Answer from the drawing. Dimensions are ordinates in mm from the lowest x, y and z of the part. A direction names the side the tool comes from. Give positions to 0.01 mm unless a question says otherwise; leave off trailing zeros. Loops run counter-clockwise (first coordinate to the right, second up) from the corner with the lowest first, then second, coordinate; pieces in that order, holes last.
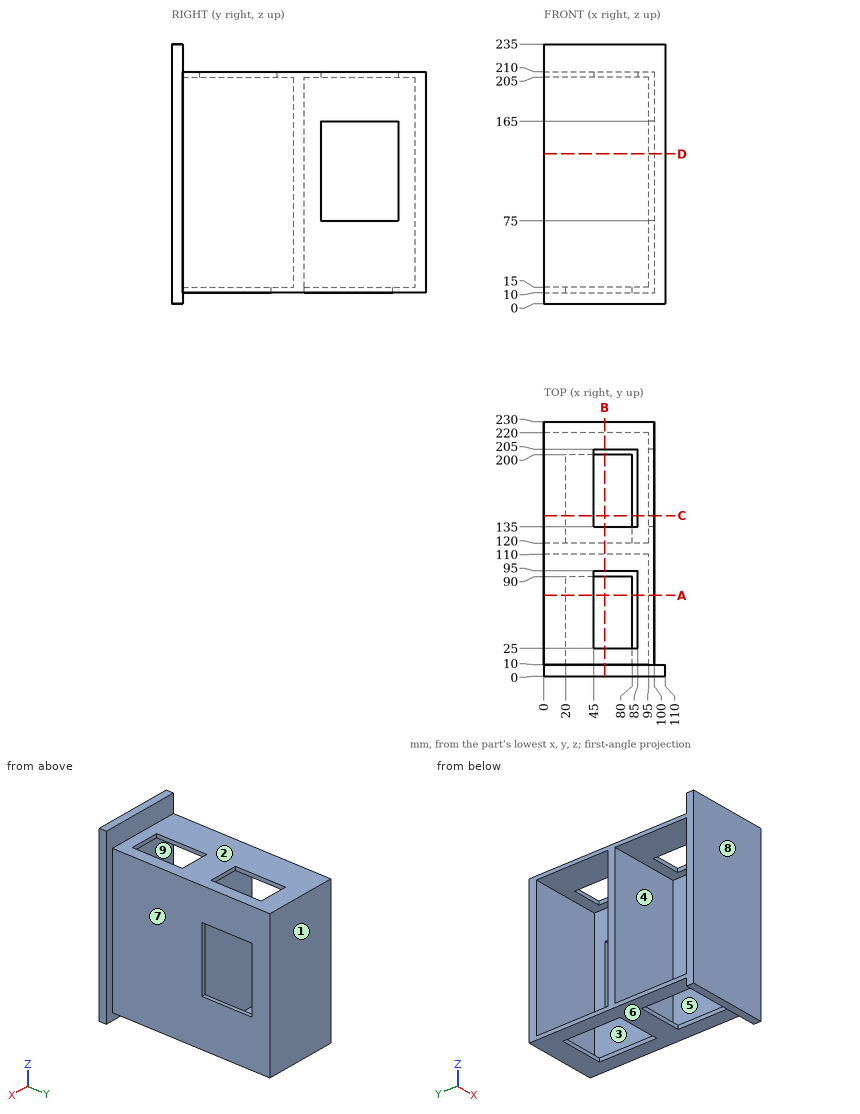
Item 1: Find section C-C, the plane y = 145. Write down the section's boundary in (x, z), plus the area to 3 significant figures.
Item 2: Find section B-B, the plane x = 55. Write down the section's boundary in (y, z), plus the area to 3 significant figures.
Item 3: Find section A-A, the plane y = 73. Write down the section's boundary in (x, z), plus the area to 3 significant figures.
Item 4: Flat-ended cylindrical pins translate along their axes: pin 1 Ø12 at (x, y) = (26.5, 40.5) entering from +Z; pin 2 Ø12 at (y, z) = (118, 210.5) entering from +X; pin 3 Ø2.5 at (x, y) = (97.5, 156) entering from -Z. Find the tip coordinate at first contact, or state that the pin passes through.
Item 5: Find section D-D, the plane z = 135.5. Write down the section's boundary in (x, y), plus the area to 3 significant figures.
Item 6: Determine the mould class of the marked faces 1, 2, 3 and 4 for opening direction Z: released by +Z, released by -Z, zero draft, split by the parting line, or undercut.
Item 7: Consider line 1 (Y direction, x = 63, z = 86.5); line 2 (Z direction, x = 6, y = 168); line 3 (Z direction, x = 98, y = 151.5). Determine where each line is inside the solid, lowest interval first.
Item 8: For the marked faces 5, 6, 7, 8 and 9, determine the directions among +Z, -Z, +X, -X, +Y, -Y from which every point of the face is accessible in a straight line to the end or side of a thin tool.
Ans:
1. outline: (0, 10) - (20, 10) - (20, 15) - (0, 15) - close; (0, 205) - (45, 205) - (45, 210) - (0, 210) - close; (80, 10) - (100, 10) - (100, 75) - (95, 75) - (95, 15) - (80, 15) - close; (85, 205) - (95, 205) - (95, 165) - (100, 165) - (100, 210) - (85, 210) - close
1. area: 1,000 mm2
2. outline: (0, 0) - (10, 0) - (10, 205) - (25, 205) - (25, 210) - (10, 210) - (10, 235) - (0, 235) - close; (90, 10) - (120, 10) - (120, 205) - (135, 205) - (135, 210) - (95, 210) - (95, 205) - (110, 205) - (110, 15) - (90, 15) - close; (200, 10) - (230, 10) - (230, 210) - (205, 210) - (205, 205) - (220, 205) - (220, 15) - (200, 15) - close
2. area: 6,850 mm2
3. outline: (0, 10) - (20, 10) - (20, 15) - (0, 15) - close; (0, 205) - (45, 205) - (45, 210) - (0, 210) - close; (80, 10) - (100, 10) - (100, 210) - (85, 210) - (85, 205) - (95, 205) - (95, 15) - (80, 15) - close
3. area: 1,450 mm2
4. pin 1: stops at z = 210
4. pin 2: stops at x = 100
4. pin 3: stops at z = 10
5. outline: (0, 0) - (110, 0) - (110, 10) - (100, 10) - (100, 135) - (95, 135) - (95, 120) - (0, 120) - (0, 110) - (95, 110) - (95, 10) - (0, 10) - close; (0, 220) - (95, 220) - (95, 205) - (100, 205) - (100, 230) - (0, 230) - close
5. area: 3,750 mm2
6. face 1: zero draft
6. face 2: released by +Z
6. face 3: undercut
6. face 4: undercut
7. line 1: y = 0 to 10, 110 to 120, 220 to 230
7. line 2: z = 10 to 15, 205 to 210
7. line 3: z = 10 to 75, 165 to 210
8. face 5: -X
8. face 6: -Z, +X, -X, +Y
8. face 7: +Z, -Z, +X, +Y
8. face 8: +Z, -Z, +X, -X, -Y
8. face 9: none
